Here's how the part is built. I have some questions about the finished solid (model axes, mm). Face numbers are marked on the shaded views. A direction names the side the tool comes from. Round coordinates to 2 decimals unless told otherwise and drop trailing zeros. Loops run counter-clockwise (first coordinate to the right, second up) from the corner with the lowest first, then second, coordinate; pieces in that order, holes last. Notation, with made-up numbers: (-31.5, 14.5) - (-6.5, 14.5) arc R26 ccw to (-6.5, 31.5) - close; hole circle Ø5 at (-39, -11.75). An arc over 180 degrees is marked (long way). Answer as a JSON object with one key per item and string values. Group by question number.
1) If I drill on line 1 along X through (y, z) = (8.25, -3.75); line 2 along X through (y, z) = (4, -7.25); line 3 along X through (y, z) = (6.75, -2), over which ranges is the centre line in solid material (lowest first)? Write a range as [from, to].
2) I want a section at C-C, the plane y = 5. Give the number of separate pieces and of enclosed holes in the cut face, then the cut area to 3 significant figures.
3) Which directions (+Z, -Z, +X, -X, +Y, -Y) give clear straight access to the entire face, cutting with the end or side of a thin tool? Please do the marked faces 1, 2 and 3.
4) I want a section at B-B, the plane x = 13.5. Please give me the cut outline in (y, z) (3 decimals), then the cut area to 3 significant figures.
5) If we mould it in two halves opening along X, with no side actions, what happens to the marked faces 4, 5, 6 and 7? For each: pulls with the +X half, pulls with the -X half, needs draft (parallel to the pull), parting line crosses it, or undercut.
6) Will these pins go through, and if not, where does the flat tip stop? P1, Ø3.5, axis at y = 4, z = -6, coming from the -X side; P2, Ø1, axis at x = 11, z = -10.5, coming from the +Y side; P3, Ø1, axis at x = 16, y = 2, coming from the -Z side.
7) I want a section at A-A, the plane z = -6.25. Please give me the cut outline in (x, y) (3 decimals).
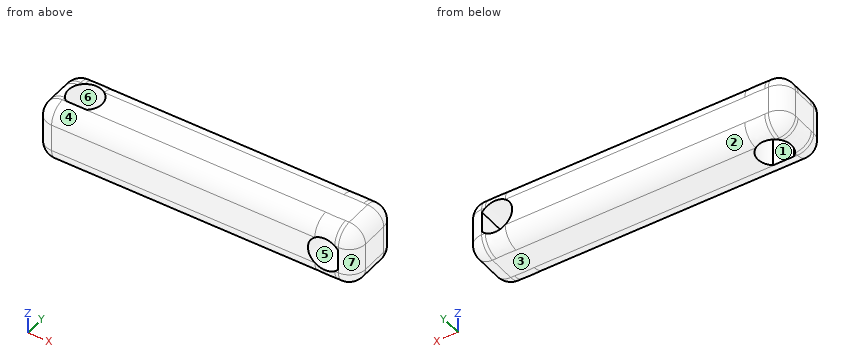
Autodesk Inventor part; units mm, degrees
ref_plane "YZ Plane" through (0, 0, 0) normal (1, 0, 0) x (0, 1, 0)
ref_plane "XZ Plane" through (0, 0, 0) normal (0, 1, 0) x (-1, 0, 0)
ref_plane "XY Plane" through (0, 0, 0) normal (0, 0, 1) x (1, 0, 0)
sketch "Sketch1" plane through (0, 0, 0) normal (0, 1, 0) x (-1, 0, 0)
  line L0 (0, 0) -> (-62.484, 0)
  line L1 (-62.484, 0) -> (-62.484, -11.684)
  line L2 (-62.484, -11.684) -> (0, -11.684)
  line L3 (0, -11.684) -> (0, 0)
  arc A0 (-59.2328, -7.8892) -> (-59.2328, -3.7948) centre (-56.642, -5.842) ccw
  line L4 (-59.2328, -3.7948) -> (-59.2328, -7.8892)
  dimension "d0" = 62.484
  dimension "d1" = 11.684
  dimension "d2" = 6.604
  dimension "d3" = 5.842
  dimension "d4" = 5.842
  dimension "d5" = 5.842
  dimension "d6" = 2.5908
extrude "Extrusion1" add sketch "Sketch1" along normal blind 11.684
sketch "Sketch3" plane through (0, 0, 0) normal (0, 0, 1) x (1, 0, 0)
  arc A0 (7.8892, 3.2512) -> (3.7948, 3.2512) centre (5.842, 5.842) ccw
  line L0 (0, 0) -> (0, 11.684)
  line L1 (0, 0) -> (62.484, 0)
  line L2 (3.7948, 3.2512) -> (7.8892, 3.2512)
  dimension "d9" = 6.604
  dimension "d10" = 5.842
  dimension "d11" = 5.842
  dimension "d12" = 2.5908
extrude "Extrusion2" cut sketch "Sketch3" against normal blind 11.684
fillet "Fillet1" radius 3.175 4 edges at (0, 11.684, -5.842) (0, 0, -5.842) (62.484, 11.684, -5.842) (62.484, 0, -5.842)
fillet "Fillet2" radius 3.175 16 edges at (61.5541, 10.7541, -11.684) (31.242, 11.684, -11.684) (0.9299, 10.7541, -11.684) (0, 5.842, -11.684) (0.9299, 0.9299, -11.684) (31.242, 0, -11.684) (61.5541, 0.9299, -11.684) (62.484, 5.842, -11.684) (61.5541, 10.7541, 0) (62.484, 5.842, 0) (61.5541, 0.9299, 0) (31.242, 0, 0) (0.9299, 0.9299, 0) (0, 5.842, 0) (0.9299, 10.7541, 0) (31.242, 11.684, 0)
properties part number "Carrier arm"
Outcome:
{
 "1": {"line 1": "[0, 3.58], [8.1, 54.09], [59.2, 62.48]", "line 2": "[0, 3.1], [8.58, 53.66], [59.23, 62.48]", "line 3": "[0.21, 2.67], [9.02, 62.26]"},
 "2": {"separate pieces": "2", "enclosed holes": "1", "area": "615 mm^2"},
 "3": {"face 1": "+Z, -Z", "face 2": "-Z, +Y", "face 3": "-Z, +X, -X, +Y, -Y"},
 "4": {"outline": "(0, -8.509) arc R3.175 ccw to (3.175, -11.684) - (8.509, -11.684) arc R3.175 ccw to (11.684, -8.509) - (11.684, -3.175) arc R3.175 ccw to (8.509, 0) - (3.175, 0) arc R3.175 ccw to (0, -3.175) - close", "area": "128 mm^2"},
 "5": {"face 4": "needs draft", "face 5": "undercut", "face 6": "undercut", "face 7": "pulls with the +X half"},
 "6": {"P1": "x = 0", "P2": "y = 11.31", "P3": "z = -11.61"},
 "7": {"outline": "(0, 3.175) arc R3.175 ccw to (3.175, 0) - (53.365, 0) - (53.365, 11.684) - (3.175, 11.684) arc R3.175 ccw to (0, 8.509) - close; (59.233, 0) - (59.309, 0) arc R3.175 ccw to (62.484, 3.175) - (62.484, 8.509) arc R3.175 ccw to (59.309, 11.684) - (59.233, 11.684) - close; hole (3.795, 3.251) - (7.889, 3.251) arc R3.302 ccw (long way) to start"}
}
